Part model, mm, in its own coordinate system. A direction names the side the tool comes from. Give positions to 0.01 mm unless a question says otherwise; leave off trailing zeros. Write each loop counter-clockwise with the first axis right and the second up, starting at its lowest first coordinate (ties: lowest second). Pieces come first, ordered by that corner, then holes. Notation, with made-up numbers: (5.5, -28.5) - (22.5, -28.5) arc R29 ccw to (22.5, -0.5) - close; hole circle Ø8 at (87, -24). An arc over 180 degrees is marked (long way). Answer in a Markdown table with one row per item. Add a question column.
1. Pull direction X, two halves, no side cores. Call faces 1 (the cylindrical face through (-2.17, 2.96, 9.76)), 2 (the flat face through (-5, 6, 2)), 3 (the flat face through (0, 3, 0)): released by +X, released by -X, zero draft, split by the parting line, or undercut.
2. Probe line 1 along Y through (x, z) = (0, 4.1); line 2 along X through (y, z) = (5, 0); line 3 along Z through (x, y) = (-6.25, 5). List the from-to ranges inside material, lowest first.
3. Band-saw the part on A-A on x = 0. Write the cut outline in (y, z).
4. Band-saw the part on D-D on z = 0. Write the cut outline in (x, y), plus the area to 4 significant figures.
5. Drop flat-ended pins along their axis: pin 1 Ø4 at (x, z) = (-5.4, 5.4) entering from +Y; pin 2 Ø4 at (x, y) = (0, 9) entering from -Z; pin 3 Ø6 at (x, y) = (2.5, 9.5) entering from +Z. Give the stop position or say it passes through.
6. Band-saw the part on C-C on x = -5.4. Write the cut outline in (y, z), plus the area to 3 significant figures.
7. Which spindle directions (+Z, -Z, +X, -X, +Y, -Y) get a long thin tool onto all of the face, cutting with end or side? Do faces 4 (the cylindrical face through (1.19, 9.38, 3.46)), 5 (the cylindrical face through (3, 9, -4)), 6 (the cylindrical face through (6.878, 3.042, -5.866)). Say none if no direction does.
8. Band-saw the part on B-B on z = -5.4. Write the cut outline in (x, y).
```python
from build123d import *

# Parameters (mm, degrees)
SKIZZE1_R                       = 10
AUFSATZ_LINEAR_AUSTRAGEN1_DEPTH = 6
SKIZZE2_R                       = 5
AUFSATZ_LINEAR_AUSTRAGEN2_DEPTH = 6
SKIZZE3_R                       = 2.25
SCHNITT_LINEAR_AUSTRAGEN1_DEPTH = 9
SKIZZE4_R                       = 1.55
SCHNITT_LINEAR_AUSTRAGEN2_DEPTH = 7
SCHNITT_LINEAR_AUSTRAGEN3_REACH = 17
SKIZZE5_R                       = 1.25


with BuildPart() as part:
    # Skizze1 → Aufsatz-Linear austragen1 (new body)
    with BuildSketch(Plane(origin=(0, 0, 0), x_dir=(1, 0, 0), z_dir=(0, 1, 0))):
        Circle(SKIZZE1_R)
    extrude(amount=AUFSATZ_LINEAR_AUSTRAGEN1_DEPTH)

    # Skizze2 → Aufsatz-Linear austragen2 (add)
    with BuildSketch(Plane(origin=(0, 6, 0), x_dir=(1, 0, 0), z_dir=(0, 1, 0))):
        Circle(SKIZZE2_R)
    extrude(amount=AUFSATZ_LINEAR_AUSTRAGEN2_DEPTH)

    # Skizze3 → Schnitt-Linear austragen1 (cut)
    with BuildSketch(Plane(origin=(0, 12, 0), x_dir=(1, 0, 0), z_dir=(0, 1, 0))):
        Circle(SKIZZE3_R)
    extrude(amount=-SCHNITT_LINEAR_AUSTRAGEN1_DEPTH, mode=Mode.SUBTRACT)

    # Skizze4 → Schnitt-Linear austragen2 (cut, through all)
    with BuildSketch(Plane(origin=(0, 6, 0), x_dir=(1, 0, 0), z_dir=(0, 1, 0))):
        with Locations((-5.4, 5.4)):
            Circle(SKIZZE4_R)
        with Locations((5.4, 5.4)):
            Circle(SKIZZE4_R)
        with Locations((5.4, -5.4)):
            Circle(SKIZZE4_R)
        with Locations((-5.4, -5.4)):
            Circle(SKIZZE4_R)
    extrude(amount=-SCHNITT_LINEAR_AUSTRAGEN2_DEPTH, mode=Mode.SUBTRACT)

    # Skizze5 → Schnitt-Linear austragen3 (cut, up to next)
    with BuildSketch(Plane.XY.offset(5), mode=Mode.PRIVATE) as schnitt_linear_austragen3_sk1:
        with Locations((0, 9)):
            Circle(SKIZZE5_R)
    schnitt_linear_austragen3_tool1 = extrude(schnitt_linear_austragen3_sk1.sketch, amount=-SCHNITT_LINEAR_AUSTRAGEN3_REACH, mode=Mode.PRIVATE) & part.part
    add(schnitt_linear_austragen3_tool1.solids().sort_by_distance((0, 9, 5))[0], mode=Mode.SUBTRACT)


solid = part.part
```
Values:
| question | item | result |
|---|---|---|
| 1 | face 1 | split by the parting line |
| 1 | face 2 | zero draft |
| 1 | face 3 | undercut |
| 2 | line 1 | y = 0 to 7.75, 10.25 to 12 |
| 2 | line 2 | x = -10 to -2.25, 2.25 to 10 |
| 2 | line 3 | z = -7.81 to -6.7, -4.1 to 4.1, 6.7 to 7.81 |
| 3 | outline | (0, -10) - (6, -10) - (6, -5) - (12, -5) - (12, -2.25) - (3, -2.25) - (3, 2.25) - (7.75, 2.25) - (7.75, 5) - (6, 5) - (6, 10) - (0, 10) - close; (10.25, 2.25) - (12, 2.25) - (12, 5) - (10.25, 5) - close |
| 4 | outline | (-10, 0) - (10, 0) - (10, 6) - (5, 6) - (5, 12) - (2.25, 12) - (2.25, 3) - (-2.25, 3) - (-2.25, 12) - (-5, 12) - (-5, 6) - (-10, 6) - close |
| 4 | area | 139.5 mm² |
| 5 | pin 1 | stops at y = 6 |
| 5 | pin 2 | stops at z = -5 |
| 5 | pin 3 | stops at z = 5 |
| 6 | outline | (0, -8.42) - (6, -8.42) - (6, -6.95) - (0, -6.95) - close; (0, -3.85) - (6, -3.85) - (6, 3.85) - (0, 3.85) - close; (0, 6.95) - (6, 6.95) - (6, 8.42) - (0, 8.42) - close |
| 6 | area | 63.8 mm² |
| 7 | face 4 | +Z |
| 7 | face 5 | +Y |
| 7 | face 6 | +Y, -Y |
| 8 | outline | (-8.42, 0) - (-6.95, 0) - (-6.95, 6) - (-8.42, 6) - close; (-3.85, 0) - (3.85, 0) - (3.85, 6) - (-3.85, 6) - close; (6.95, 0) - (8.42, 0) - (8.42, 6) - (6.95, 6) - close |
